Work out the finished part from the listing and answer in its coordinate system (mm). A direction names the side the tool comes from. Coordinates: 2 decimals unless noted, no trailing zeros. Write each loop counter-clockwise with the first axis right and the second up, starting at its lowest first coordinate (ties: lowest second). Pieces come first, ordered by that corner, then holes. Notation, with made-up numbers: M 25.5,-25 L 37.5,-25 A23 ccw 37.5,2 Z; hole C 19,58 d9. An arc over 180 degrees is marked long. Use CSV: the item, a comma, the result in double quotes.
Autodesk Inventor part; units mm, degrees
ref_plane "YZ Plane" through (0, 0, 0) normal (1, 0, 0) x (0, 1, 0)
ref_plane "XZ Plane" through (0, 0, 0) normal (0, 1, 0) x (-1, 0, 0)
ref_plane "XY Plane" through (0, 0, 0) normal (0, 0, 1) x (1, 0, 0)
sketch "Эскиз1" plane through (0, 0, 0) normal (0, 1, 0) x (-1, 0, 0)
  line L0 (13, 16) -> (-13, 16)
  line L1 (-16, 13) -> (-16, -13)
  line L2 (-13, -16) -> (13, -16)
  line L3 (16, -13) -> (16, 13)
  line L4 (0, 0) -> (32.4367, 0) construction
  line L5 (0, 0) -> (0, -34.7046) construction
  circle A0 centre (13.4, -13.4) radius 1.625
  circle A1 centre (-13.4, -13.4) radius 1.625
  circle A2 centre (13.4, 13.4) radius 1.625
  circle A3 centre (-13.4, 13.4) radius 1.625
  arc A4 (16, 13) -> (13, 16) centre (13, 13) ccw
  arc A5 (13, -16) -> (16, -13) centre (13, -13) ccw
  arc A6 (-16, -13) -> (-13, -16) centre (-13, -13) ccw
  arc A7 (-13, 16) -> (-16, 13) centre (-13, 13) ccw
  point P0 (-16, -16)
  point P1 (-16, 16)
  point P2 (16, -16)
  dimension "d0" = 32
  dimension "d1" = 32
  dimension "d2" = 3.25
  dimension "d3" = 26.8
  dimension "d4" = 26.8
  dimension "d5" = 3
extrude "Выдавливание1" add sketch "Эскиз1" along normal blind 1.6
sketch "Эскиз2" plane through (0, 1.6, 0) normal (0, 1, 0) x (1, 0, 0)
  line L0 (-10.4, 13.6) -> (-0.1, 13.6)
  line L1 (-0.1, 13.6) -> (-0.1, 16)
  line L2 (-0.1, 16) -> (-10.4, 16)
  line L3 (-10.4, 16) -> (-10.4, 13.6)
  line L4 (-13, -16) -> (13, -16) construction
  arc A0 (13, -16) -> (16, -13) centre (13, -13) ccw construction
  line L5 (16, -13) -> (16, 13) construction
  arc A1 (16, 13) -> (13, 16) centre (13, 13) ccw construction
  line L6 (13, 16) -> (-13, 16) construction
  arc A2 (-13, 16) -> (-16, 13) centre (-13, 13) ccw construction
  line L7 (-16, 13) -> (-16, -13) construction
  arc A3 (-16, -13) -> (-13, -16) centre (-13, -13) ccw construction
  circle A4 centre (13.4, 13.4) radius 1.625 construction
  circle A5 centre (13.4, -13.4) radius 1.625 construction
  circle A6 centre (-13.4, -13.4) radius 1.625 construction
  circle A7 centre (-13.4, 13.4) radius 1.625 construction
  point P0 (0, 0)
  dimension "d8" = 10.3
  dimension "d9" = 2.4
  dimension "d10" = 5.6
extrude "Выдавливание2" add sketch "Эскиз2" along normal blind 10
sketch "Эскиз3" plane through (0, 0, 0) normal (0, -1, 0) x (1, 0, 0)
  line L0 (16.3, 9.4) -> (9.3, 9.4)
  line L1 (9.3, 9.4) -> (9.3, 1.6)
  line L2 (9.3, 1.6) -> (16.3, 1.6)
  line L3 (16.3, 1.6) -> (16.3, 9.4)
  line L4 (-13, 16) -> (13, 16) construction
  arc A0 (-13, 16) -> (-16, 13) centre (-13, 13) ccw construction
  line L5 (-16, -13) -> (-16, 13) construction
  arc A1 (-16, -13) -> (-13, -16) centre (-13, -13) ccw construction
  line L6 (13, -16) -> (-13, -16) construction
  arc A2 (13, -16) -> (16, -13) centre (13, -13) ccw construction
  line L7 (16, 13) -> (16, -13) construction
  arc A3 (16, 13) -> (13, 16) centre (13, 13) ccw construction
  circle A4 centre (13.4, -13.4) radius 1.625 construction
  circle A5 centre (13.4, 13.4) radius 1.625 construction
  circle A6 centre (-13.4, 13.4) radius 1.625 construction
  circle A7 centre (-13.4, -13.4) radius 1.625 construction
  point P0 (0, 0)
  dimension "d13" = 0.3
  dimension "d14" = 7.8
  dimension "d15" = 7
  dimension "d16" = 6.6
extrude "Выдавливание3" add sketch "Эскиз3" along normal blind 3
properties part number "razor_sketch"
Item 1: The part is cut by section C-C (y = 2). Write down the section's boundary in (x, z).
Answer:
outline,"M -10.4,-16 L -0.1,-16 L -0.1,-13.6 L -10.4,-13.6 Z"
Item 2: The part is cut by section A-A (x = 13.4). Write down the section's boundary in (y, z) (3 decimals), then the cut area to 3 significant figures.
Answer:
outline,"M -3,1.6 L 0,1.6 L 0,-11.775 L 1.6,-11.775 L 1.6,11.775 L 0,11.775 L 0,9.4 L -3,9.4 Z; M 0,-15.973 L 1.6,-15.973 L 1.6,-15.025 L 0,-15.025 Z; M 0,15.025 L 1.6,15.025 L 1.6,15.973 L 0,15.973 Z"
area,"64.1 mm2"
Item 3: For a pull along Z with two mould halves and no side action, classify faces 1 (the face through (13.61, 0.79, 11.79)), 2 (the face through (0, 1.6, 0)), 3 (the face through (-5, 7, -13.6)) as released by +Z, released by -Z, zero draft, split by the parting line, or undercut.
Answer:
face 1,"undercut"
face 2,"zero draft"
face 3,"released by +Z"
Item 4: Given pin 1 (0.7 mm diameter, centred on y = 8.5, z = -15, fed in from +X); pin 2 (5 mm diameter, centred on x = -13.4, z = -13.4, fed in from +Y); pin 3 (8 mm diameter, centred on x = -4.5, y = 9, fed in from +Z), each flat-ended and moving along its own axis, determine where each tip first touches the part or whether it passes through.
Answer:
pin 1,"stops at x = -0.1"
pin 2,"stops at y = 1.6"
pin 3,"stops at z = -13.6"
Item 5: A tool of negligible diameter and unlimited length cuts with its end or side. For faces 4 (the face through (0, 1, 16)), 5 (the face through (9.3, -1, 6)), 6 (the face through (16, 1, 0)), from which of +Z, -Z, +X, -X, +Y, -Y can it reach the whole face along a straight path? Write none if from no direction.
Answer:
face 4,"+Z, +X, -X, +Y, -Y"
face 5,"+Z, -Z, -X, -Y"
face 6,"+Z, -Z, +X, +Y"
Item 6: The part is cut by section B-B (z = 13.4). Write down the section's boundary in (x, y) (3 decimals), then the cut area to 3 significant figures.
Answer:
outline,"M -15.973,0 L -15.025,0 L -15.025,1.6 L -15.973,1.6 Z; M -11.775,0 L 11.775,0 L 11.775,1.6 L -11.775,1.6 Z; M 15.025,0 L 15.973,0 L 15.973,1.6 L 15.025,1.6 Z"
area,"40.7 mm2"
Item 7: The part is cut by section D-D (z = -6). Write down the section's boundary in (x, y).
Answer:
outline,"M -16,0 L 16,0 L 16,1.6 L -16,1.6 Z"
Item 8: Consider probe 1 along X at (y, z) = (0.25, -12.5); probe 2 along Z at (x, y) = (-13.4, 0.4) (3 decimals); probe 3 along Z at (x, y) = (12, -1.25). Determine where each line is inside the solid, lowest interval first.
Answer:
probe 1,"x = -16 to -14.75, -12.05 to 12.05, 14.75 to 16"
probe 2,"z = -15.973 to -15.025, -11.775 to 11.775, 15.025 to 15.973"
probe 3,"z = 1.6 to 9.4"
